Study the drawing (mm; zero at the part's minimum x, y, z) and answer. A direction names the side the tool comes from. Round coordinates to 2 decimals unless told otherwise and drop trailing zeros. Write each loop counter-clockwise with the first axis right and the second up, starting at its lowest first coordinate (ties: lowest second). Pieces come first, ordered by that corner, then holes.
(1) Each of these flat-tipped pins is pushed along its axis until it touches: pin 1 Ø2 at (y, z) = (3.5, 2.5) entering from -X (1 decimal); pin 2 Ø4 at (x, y) = (10.5, 15.5) entering from +Z; pin 3 Ø2 at (x, z) = (21.5, 4.5) entering from -Y. Where does it stop, or does it pass through?
(2) For the marked faces 1, 2 and 3, determine the directions among +Z, -Z, +X, -X, +Y, -Y from which every point of the face is accessible in a straight line to the end or side of a thin tool.
(3) The mould has two halves that part along Z. Classify the marked faces 4, 5 and 6: +Z half, -Z half, draft (parallel to the pull), parting line (faces both ways), or undercut.
(4) Find the intervals of material crossed by probe 1 along Z at (x, y) = (2.05, 10.8) (1 decimal); probe 2 along Y at (x, z) = (11.5, 6.25); probe 3 along X at (y, z) = (5.25, 4.25) (1 decimal), in increasing order.
(5) A cutting plane is placed at C-C, the plane y = 14.25. Give the vertices of the cut face in (x, z).
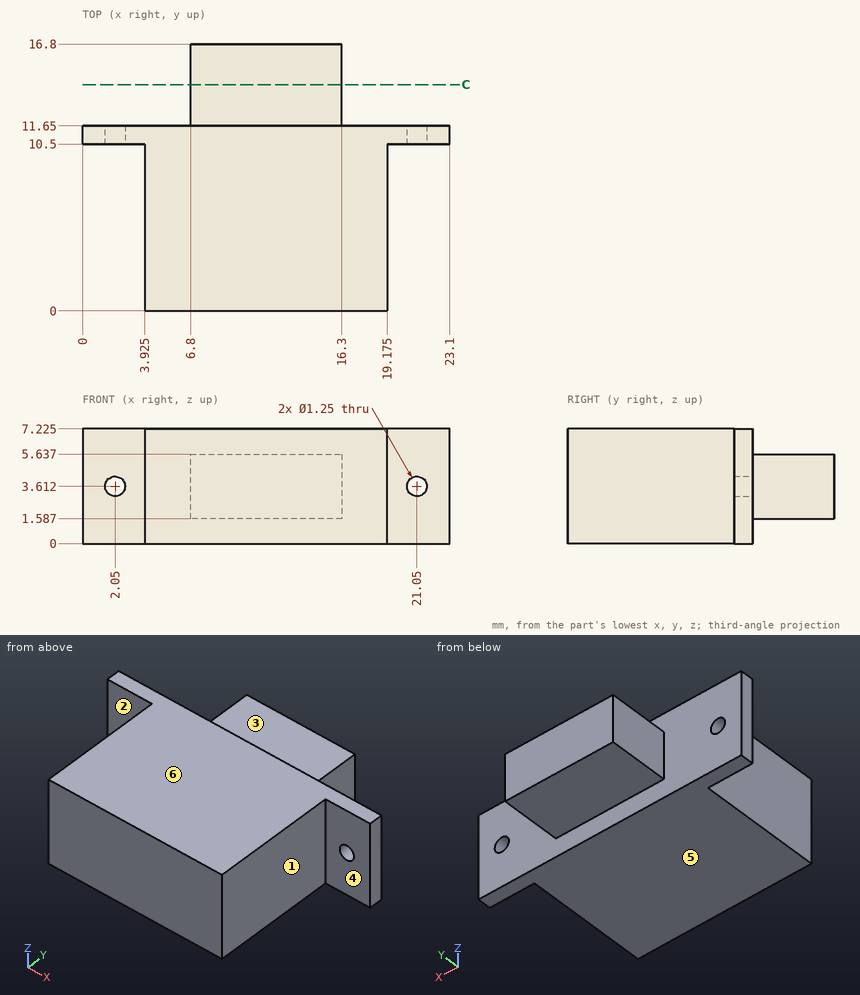
Solutions:
1. pin 1: stops at x = 3.9
1. pin 2: stops at z = 5.64
1. pin 3: stops at y = 10.5
2. face 1: +Z, -Z, +X, -Y
2. face 2: +Z, -Z, -X, -Y
2. face 3: +Z, +X, -X, +Y
3. face 4: draft
3. face 5: -Z half
3. face 6: +Z half
4. probe 1: z = 0 to 3, 4.2 to 7.2
4. probe 2: y = 0 to 11.65
4. probe 3: x = 3.9 to 19.2
5. outline: (6.8, 1.59) - (16.3, 1.59) - (16.3, 5.64) - (6.8, 5.64) - close
